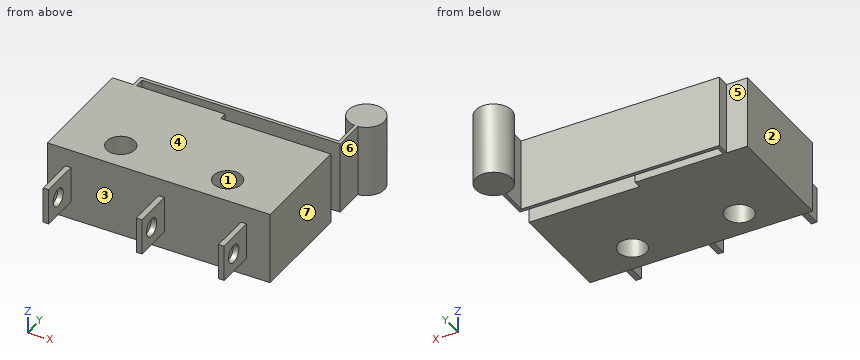
```python
from build123d import *

# Parameters (mm, degrees)
SKETCH1_R           = 1.25
BOSS_EXTRUDE1_DEPTH = 6.4
SKETCH2_W           = 0.5
SKETCH2_H           = 3.2
BOSS_EXTRUDE2_DEPTH = 3.5
CUT_EXTRUDE1_REACH  = 27.362
SKETCH3_R           = 0.8


with BuildPart() as part:
    # Sketch1 → Boss-Extrude1 (new body)
    with BuildSketch(Plane.XY):
        with BuildLine():
            Line((0, 0), (19.8, 0))
            Line((19.8, 0), (19.8, 9.5))
            Line((19.8, 9.5), (10, 9.5))
            Line((10, 9.5), (10, 10.2))
            Line((10, 10.2), (2.15, 10.2))
            Line((2.15, 10.2), (2.15, 11.05))
            Line((2.15, 11.05), (19.75, 11.05))
            Line((19.75, 11.05), (19.75, 13.807046768))
            ThreePointArc((19.75, 13.807046768), (19.6, 17), (19.45, 13.807046768))
            Line((19.45, 13.807046768), (19.45, 11.35))
            Line((19.45, 11.35), (1.85, 11.35))
            Line((1.85, 11.35), (1.85, 10.2))
            Line((1.85, 10.2), (0, 10.2))
            Line((0, 10.2), (0, 4.415474079))
            Line((0, 4.415474079), (0, 0))
        make_face()
        with Locations((14.6, 2.5)):
            Circle(SKETCH1_R, mode=Mode.SUBTRACT)
        with Locations((5.1, 2.5)):
            Circle(SKETCH1_R, mode=Mode.SUBTRACT)
    extrude(amount=BOSS_EXTRUDE1_DEPTH)

    # Sketch2 → Boss-Extrude2 (add)
    with BuildSketch(Plane.XZ):
        with Locations((1.85, 3.2)):
            Rectangle(SKETCH2_W, SKETCH2_H)
        with Locations((10.15, 3.2)):
            Rectangle(SKETCH2_W, SKETCH2_H)
        with Locations((17.45, 3.2)):
            Rectangle(SKETCH2_W, SKETCH2_H)
    extrude(amount=BOSS_EXTRUDE2_DEPTH)

    # Cut-Extrude1: up to this face of the body (flat: up to its plane)
    cut_extrude1_end = Plane(part.part.faces().sort_by_distance((1.6, -1.75, 3.2))[0])
    # Sketch3 → Cut-Extrude1 (cut, up to the picked face)
    with BuildSketch(Plane(origin=(17.7, 0, 0), x_dir=(0, 0, -1), z_dir=(1, 0, 0)), mode=Mode.PRIVATE) as cut_extrude1_sk1:
        with Locations((-3.2, -2)):
            Circle(SKETCH3_R)
    cut_extrude1_tool1 = split(extrude(cut_extrude1_sk1.sketch, amount=-CUT_EXTRUDE1_REACH, mode=Mode.PRIVATE), bisect_by=cut_extrude1_end, keep=Keep.BOTH, mode=Mode.PRIVATE)
    add(cut_extrude1_tool1.solids().sort_by(Axis((17.7, -2, 3.2), (-1, 0, 0)))[0], mode=Mode.SUBTRACT)


solid = part.part
```
Verification items for the finished model (mm, model axes). Face numbers are marked on the shaded views. A direction names the side the tool comes from. Give positions to 0.01 mm unless a question says otherwise; leave off trailing zeros. Order: outer loops, then holes, each group sorted by start corner. A loop starts at its lowest first (then second) coordinate and runs counter-clockwise, first axis right, second up. Notation, with made-up numbers: (5, 76.25) -> (21, 76.25) arc R14 ccw to (21, 102.25) -> close; hole circle Ø9 at (-11.5, 49). An arc over 180 degrees is marked (long way). Use a Markdown table: item, result.
1) Mould release check, pull along X, two halves, no side actions. Record for the marked faces 1, 2, 3 and 4: pulls with the +X half, pulls with the -X half, needs draft (parallel to the pull), parting line crosses it, or undercut.
Results:
| item | result |
|---|---|
| face 1 | undercut |
| face 2 | pulls with the -X half |
| face 3 | undercut |
| face 4 | needs draft |
2) Tool access check on the marked faces 5, 6 and 7. Record the directions out of +Z, -Z, +X, -X, +Y, -Y that give a thin tool (end or side, any length) a straight path to the whole face; none if there is none.
Results:
| item | result |
|---|---|
| face 5 | +Z, -Z, -X, +Y |
| face 6 | +Z, -Z, +X |
| face 7 | +Z, -Z, +X, -Y |
3) Material ranges on probe 1 along Y at (x, z) = (10.3, 3.2); probe 2 along Y at (x, z) = (5.1, 2); probe 3 along Y at (x, z) = (12.25, 3.5), recorded low to high.
Results:
| item | result |
|---|---|
| probe 1 | -3.5 to -2.8, -1.2 to 9.5, 11.05 to 11.35 |
| probe 2 | 0 to 1.25, 3.75 to 10.2, 11.05 to 11.35 |
| probe 3 | 0 to 9.5, 11.05 to 11.35 |
4) Section check C-C, the plane x = 5.1. Record the boundary of the cut face in (y, z).
Results:
| item | result |
|---|---|
| outline | (0, 0) -> (1.25, 0) -> (1.25, 6.4) -> (0, 6.4) -> close; (3.75, 0) -> (10.2, 0) -> (10.2, 6.4) -> (3.75, 6.4) -> close; (11.05, 0) -> (11.35, 0) -> (11.35, 6.4) -> (11.05, 6.4) -> close |
5) Section check A-A, the plane y = -2. Record the boundary of the cut face in (x, z).
Results:
| item | result |
|---|---|
| outline | (1.6, 1.6) -> (2.1, 1.6) -> (2.1, 2.4) -> (1.6, 2.4) -> close; (1.6, 4) -> (2.1, 4) -> (2.1, 4.8) -> (1.6, 4.8) -> close; (9.9, 1.6) -> (10.4, 1.6) -> (10.4, 2.4) -> (9.9, 2.4) -> close; (9.9, 4) -> (10.4, 4) -> (10.4, 4.8) -> (9.9, 4.8) -> close; (17.2, 1.6) -> (17.7, 1.6) -> (17.7, 2.4) -> (17.2, 2.4) -> close; (17.2, 4) -> (17.7, 4) -> (17.7, 4.8) -> (17.2, 4.8) -> close |
6) Section check B-B, the plane z = 2. Record the boundary of the cut face in (x, y).
Results:
| item | result |
|---|---|
| outline | (0, 0) -> (1.6, 0) -> (1.6, -3.5) -> (2.1, -3.5) -> (2.1, 0) -> (9.9, 0) -> (9.9, -3.5) -> (10.4, -3.5) -> (10.4, 0) -> (17.2, 0) -> (17.2, -3.5) -> (17.7, -3.5) -> (17.7, 0) -> (19.8, 0) -> (19.8, 9.5) -> (10, 9.5) -> (10, 10.2) -> (2.15, 10.2) -> (2.15, 11.05) -> (19.75, 11.05) -> (19.75, 13.81) arc R1.6 ccw (long way) to (19.45, 13.81) -> (19.45, 11.35) -> (1.85, 11.35) -> (1.85, 10.2) -> (0, 10.2) -> close; hole circle Ø2.5 at (5.1, 2.5); hole circle Ø2.5 at (14.6, 2.5) |
7) Depth check by flat-ended pin: pin 1 Ø1.6 at (y, z) = (-2.5, 3) entering from -X; pin 2 Ø1.5 at (x, z) = (12.5, 5.5) entering from +Y; pin 3 Ø2 at (y, z) = (9, 3.5) entering from -X; pin 4 Ø2.5 at (y, z) = (-2, 3.5) entering from +X. Enter the tip coordinate at first touch or a pass-through.
Results:
| item | result |
|---|---|
| pin 1 | x = 1.6 |
| pin 2 | y = 11.35 |
| pin 3 | x = 0 |
| pin 4 | x = 17.7 |
8) Section check D-D, the plane x = 11.25. Record the boundary of the cut face in (y, z).
Results:
| item | result |
|---|---|
| outline | (0, 0) -> (9.5, 0) -> (9.5, 6.4) -> (0, 6.4) -> close; (11.05, 0) -> (11.35, 0) -> (11.35, 6.4) -> (11.05, 6.4) -> close |
